Answer from the drawing. Dimensions are ordinates in mm from the lowest x, y and z of the part. Coordinates: 2 decimals unless noted, no trailing zeros. Loops run counter-clockwise (first coordinate to the right, second up) from the corner with the lowest first, then second, coordinate; pieces in that order, holes last.
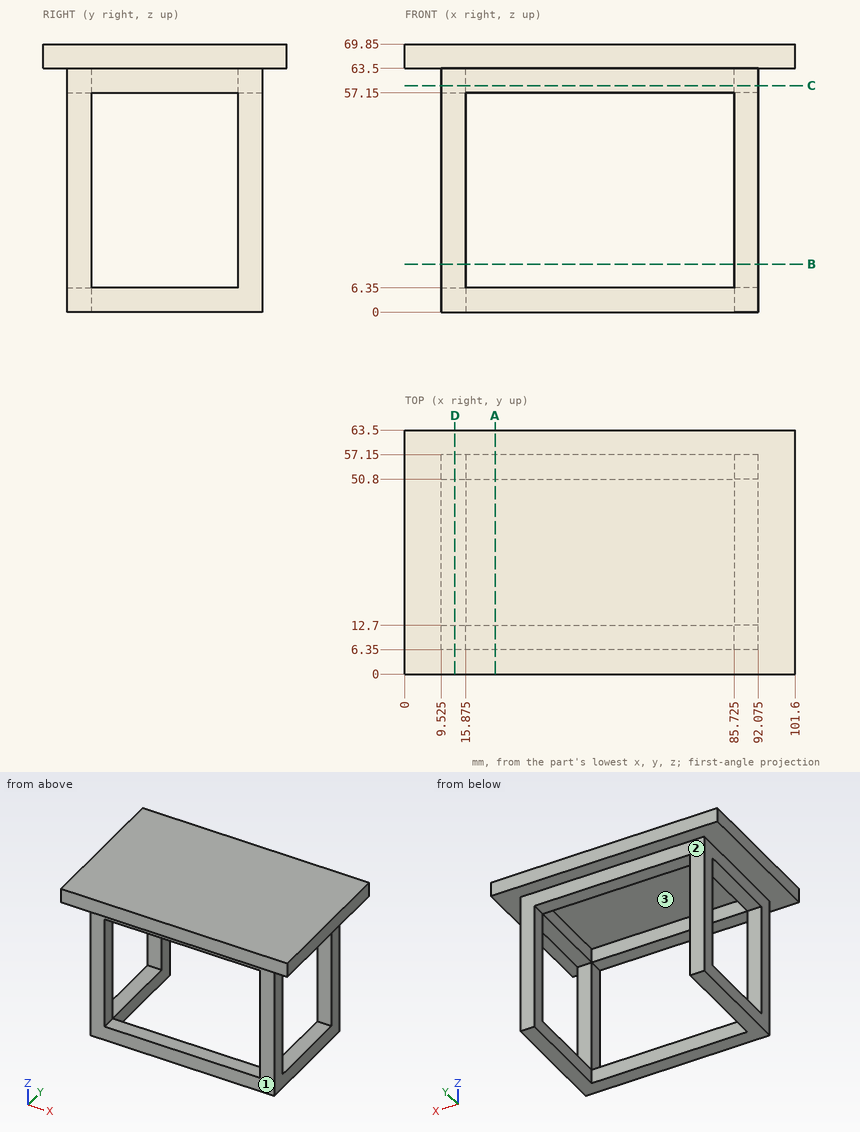
Item 1: A cutting plane is placed at D-D on x = 13. Determine the outline of the cut face in (y, z).
Numbers:
outline: (0, 63.5) - (6.35, 63.5) - (6.35, 0) - (57.15, 0) - (57.15, 63.5) - (63.5, 63.5) - (63.5, 69.85) - (0, 69.85) - close; hole (12.7, 6.35) - (50.8, 6.35) - (50.8, 57.15) - (12.7, 57.15) - close
Item 2: A cutting plane is placed at A-A on x = 23.5. Determine the outline of the cut face in (y, z).
Numbers:
outline: (0, 63.5) - (6.35, 63.5) - (6.35, 57.15) - (12.7, 57.15) - (12.7, 63.5) - (50.8, 63.5) - (50.8, 57.15) - (57.15, 57.15) - (57.15, 63.5) - (63.5, 63.5) - (63.5, 69.85) - (0, 69.85) - close; (6.35, 0) - (12.7, 0) - (12.7, 6.35) - (6.35, 6.35) - close
Item 3: Find the intervals of material crossed by line 1 along X through (y, z) = (56, 17.5) (3 decimals); line 2 along Y through (x, z) = (10.5, 36); line 3 along Z through (x, y) = (22, 9.5), in increasing order.
Numbers:
line 1: x = 9.525 to 15.875, 85.725 to 92.075
line 2: y = 6.35 to 12.7, 50.8 to 57.15
line 3: z = 0 to 6.35, 57.15 to 69.85
Item 4: A cutting plane is placed at C-C on z = 59. Determine the outline of the cut face in (x, y) (3 decimals).
Numbers:
outline: (9.525, 6.35) - (92.075, 6.35) - (92.075, 57.15) - (9.525, 57.15) - close; hole (15.875, 12.7) - (85.725, 12.7) - (85.725, 50.8) - (15.875, 50.8) - close
Item 5: Determine the mould class of the marked faces 1, 2 and 3 for opening direction Y: released by +Y, released by -Y, zero draft, split by the parting line, or undercut.
Numbers:
face 1: released by -Y
face 2: released by +Y
face 3: undercut
Item 6: Given pin 1 (5 mm diameter, centred on x = 87.5, y = 22.5, fed in from -Z); pin 2 (3 mm diameter, centred on x = 48, z = 61, fed in from +Y); pin 3 (4 mm diameter, centred on x = 81, y = 34.5, fed in from -Z); pin 4 (5 mm diameter, centred on y = 8, z = 20.5, fed in from -X) (3 decimals), each flat-ended and moving along its own axis, determine where each tip first touches the part or whether it passes through.
Numbers:
pin 1: stops at z = 0
pin 2: stops at y = 57.15
pin 3: stops at z = 63.5
pin 4: stops at x = 9.525
Item 7: A cutting plane is placed at B-B on z = 12.5. Determine the outline of the cut face in (x, y) (3 decimals).
Numbers:
outline: (9.525, 6.35) - (15.875, 6.35) - (15.875, 12.7) - (9.525, 12.7) - close; (9.525, 50.8) - (15.875, 50.8) - (15.875, 57.15) - (9.525, 57.15) - close; (85.725, 6.35) - (92.075, 6.35) - (92.075, 12.7) - (85.725, 12.7) - close; (85.725, 50.8) - (92.075, 50.8) - (92.075, 57.15) - (85.725, 57.15) - close
